Input: part model. Units: mm. Frame: model coordinates. Round coordinates to 2 decimals unless told otherwise and drop trailing zeros. Order: outer loops, then holes, each group sorted by start corner. A loop starts at its lowest first (then second) coordinate and runs counter-clockwise, first axis right, second up.
Item 1: Cut plane B-B on y = 65. Output: boundary loops of the cut face in (x, z) (1 decimal), then the cut area to 3 significant figures.
Item 2: Line query: L1, parallel to X at y = 69.5, z = 1.15 (3 decimals). Output: solid intervals per line, ascending.
Item 3: Cut plane A-A on z = 0.1. Output: boundary loops of the cut face in (x, y) (3 decimals), then the cut area to 3 significant figures.
Item 4: First-contact query: pin 1 (0.9 mm diameter, centred on y = 55, z = -0.5, fed in from -X) (3 decimals). Flat tip, straight axial feed; report the tip coordinate or a pass-through.
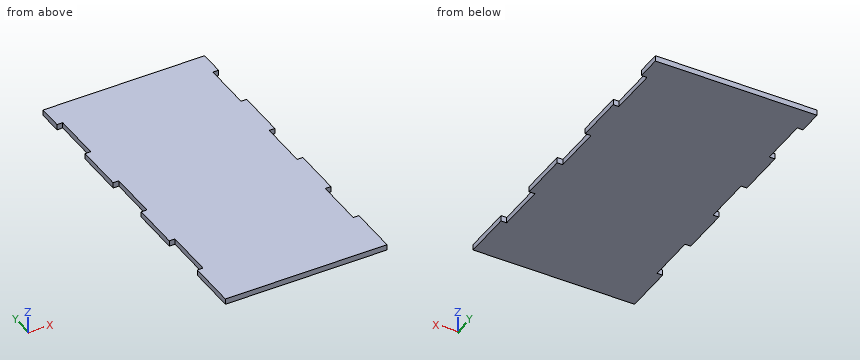
```python
from build123d import *

# Parameters (mm, degrees)
SKETCH1_W           = 83.312
SKETCH1_H           = 165.1
BOSS_EXTRUDE1_DEPTH = 1.4605
SKETCH2_W           = 2.921
SKETCH2_H           = 25.4
CUT_EXTRUDE1_DEPTH  = 2.921


with BuildPart() as part:
    # Sketch1 → Boss-Extrude1 (new, symmetric)
    with BuildSketch(Plane.XY):
        Rectangle(SKETCH1_W, SKETCH1_H)
    extrude(amount=BOSS_EXTRUDE1_DEPTH, both=True)

    # Sketch2 → Cut-Extrude1 (cut)
    with BuildSketch(Plane.XY.offset(1.4605)):
        with Locations((-40.1955, 57.15)):
            Rectangle(SKETCH2_W, SKETCH2_H)
        with Locations((-40.1955, 6.35)):
            Rectangle(SKETCH2_W, SKETCH2_H)
        with Locations((-40.1955, -44.45)):
            Rectangle(SKETCH2_W, SKETCH2_H)
        with Locations((40.1955, -44.45)):
            Rectangle(SKETCH2_W, SKETCH2_H)
        with Locations((40.1955, 6.35)):
            Rectangle(SKETCH2_W, SKETCH2_H)
        with Locations((40.1955, 57.15)):
            Rectangle(SKETCH2_W, SKETCH2_H)
    extrude(amount=-CUT_EXTRUDE1_DEPTH, mode=Mode.SUBTRACT)


solid = part.part
```
From the geometry:
1. outline: (-38.7, -1.5) - (38.7, -1.5) - (38.7, 1.5) - (-38.7, 1.5) - close
1. area: 226 mm2
2. L1: x = -38.735 to 38.735
3. outline: (-41.656, -82.55) - (41.656, -82.55) - (41.656, -57.15) - (38.735, -57.15) - (38.735, -31.75) - (41.656, -31.75) - (41.656, -6.35) - (38.735, -6.35) - (38.735, 19.05) - (41.656, 19.05) - (41.656, 44.45) - (38.735, 44.45) - (38.735, 69.85) - (41.656, 69.85) - (41.656, 82.55) - (-41.656, 82.55) - (-41.656, 69.85) - (-38.735, 69.85) - (-38.735, 44.45) - (-41.656, 44.45) - (-41.656, 19.05) - (-38.735, 19.05) - (-38.735, -6.35) - (-41.656, -6.35) - (-41.656, -31.75) - (-38.735, -31.75) - (-38.735, -57.15) - (-41.656, -57.15) - close
3. area: 13,300 mm2
4. pin 1: stops at x = -38.735
